```python
from build123d import *
from OCP.BRepAlgoAPI import BRepAlgoAPI_Cut
from OCP.TopTools import TopTools_ListOfShape

# Parameters (mm, degrees)
SKETCH1_W               = 193.19
SKETCH1_H               = 93.85
BOSS_EXTRUDE1_DEPTH     = 32.179999902
SKETCH3_W               = 93.85
SKETCH3_H               = 28.999999912
CUT_EXTRUDE1_DEPTH      = 27.67
SKETCH5_W               = 137.85
SKETCH5_H               = 32.179999902
BOSS_EXTRUDE2_DEPTH     = 12.5
SKETCH6_W               = 32
SKETCH6_H               = 40
CUT_EXTRUDE2_DEPTH      = 118.887561022
SKETCH21_W              = 116.85
SKETCH21_H              = 73.85
CUT_EXTRUDE3_DEPTH      = 118.887561022
CUT_EXTRUDE5_DEPTH      = 118.887561022
CUT_EXTRUDE5_DEPTH_BACK = 29
SKETCH22_W              = 130.49
SKETCH22_H              = 91.75
SKETCH23_W              = 130.49
SKETCH23_H              = 3.18
BOSS_EXTRUDE4_DEPTH     = 6.35
SKETCH25_R              = 2.185
CUT_EXTRUDE6_DEPTH      = 118.887561022
SKETCH26_R              = 2.185
CUT_EXTRUDE8_DEPTH      = 179.78409722
FILLET3_R               = 1
FILLET1_R               = 7.75
FILLET2_R               = 10
CUT_EXTRUDE9_REACH      = 149.229
SKETCH47_R              = 3.5
BOSS_EXTRUDE5_DEPTH     = 8
SKETCH48_R              = 3
CUT_EXTRUDE18_DEPTH     = 6
SKETCH49_R              = 3
CUT_EXTRUDE19_DEPTH     = 5
SKETCH51_R              = 3.5
BOSS_EXTRUDE6_DEPTH     = 8
SKETCH52_R              = 3
CUT_EXTRUDE21_DEPTH     = 5
SKETCH53_W              = 25.1
SKETCH53_H              = 21.647882291
SKETCH53_W_2            = 16.257833485
BOSS_EXTRUDE7_DEPTH     = 3.82
FILLET4_DEPTH           = 21.647882291
FILLET4_START           = -51.344578607
FILLET4_2_DEPTH         = 27.019578607
FILLET4_START_2         = 23.245
FILLET4_3_DEPTH         = 20.253781432
FILLET4_START_3         = 21.647882291
FILLET4_4_DEPTH         = 3.995947947
FILLET4_5_DEPTH         = 10.532117611
SKETCH54_W              = 36.508182433
SKETCH54_H              = 14.6
CUT_EXTRUDE24_DEPTH     = 22.649999902
SKETCH55_W              = 81.374829932
SKETCH55_H              = 14.6
CUT_EXTRUDE26_DEPTH     = 18
SKETCH57_W              = 36.508182433
SKETCH57_H              = 14.6
BOSS_EXTRUDE8_DEPTH     = 4.649999902


with BuildPart() as part:
    # Sketch1 → Boss-Extrude1 (new body)
    with BuildSketch(Plane(origin=(0, 0, 0), x_dir=(1, 0, 0), z_dir=(0, 1, 0))):
        Rectangle(SKETCH1_W, SKETCH1_H)
    extrude(amount=BOSS_EXTRUDE1_DEPTH)

    # Sketch3 → Cut-Extrude1 (cut)
    with BuildSketch(Plane.ZY.offset(96.595)):
        with Locations((0, 14.499999956)):
            Rectangle(SKETCH3_W, SKETCH3_H)
    cut_extrude1 = extrude(amount=-CUT_EXTRUDE1_DEPTH, mode=Mode.SUBTRACT)

    # Mirror1: Cut-Extrude1 across plane
    add(cut_extrude1.mirror(Plane(origin=(0, 0, 0), x_dir=(0, 0, 1), z_dir=(1, 0, 0))), mode=Mode.SUBTRACT)

    # Sketch5 → Boss-Extrude2 (add)
    with BuildSketch(Plane(origin=(0, 0, -46.925), x_dir=(-1, 0, 0), z_dir=(0, 0, -1))):
        with Locations((0, 16.089999951)):
            Rectangle(SKETCH5_W, SKETCH5_H)
    extrude(amount=BOSS_EXTRUDE2_DEPTH)

    # Sketch6 → Cut-Extrude2 (cut, through all)
    with BuildSketch(Plane(origin=(0, 32.179999902, 0), x_dir=(1, 0, 0), z_dir=(0, 1, 0))):
        with Locations((0, 34.425)):
            Rectangle(SKETCH6_W, SKETCH6_H)
    extrude(amount=-CUT_EXTRUDE2_DEPTH, mode=Mode.SUBTRACT)

    # Sketch21 → Cut-Extrude3 (cut, through all)
    with BuildSketch(Plane(origin=(0, 32.179999902, 0), x_dir=(1, 0, 0), z_dir=(0, 1, 0))):
        with Locations((0.5, 0)):
            Rectangle(SKETCH21_W, SKETCH21_H)
    extrude(amount=-CUT_EXTRUDE3_DEPTH, mode=Mode.SUBTRACT)

    # Sketch22 → Cut-Extrude5 (cut, two sides: drawn at the far end of the back side and taken through both)
    with BuildSketch(Plane(origin=(0, 32.179999902, 0), x_dir=(1, 0, 0), z_dir=(0, 1, 0)).offset(-CUT_EXTRUDE5_DEPTH_BACK)):
        with Locations((0.5, -1.05)):
            Rectangle(SKETCH22_W, SKETCH22_H)
    extrude(amount=CUT_EXTRUDE5_DEPTH + CUT_EXTRUDE5_DEPTH_BACK, mode=Mode.SUBTRACT)

    # Sketch23 → Boss-Extrude4 (add)
    with BuildSketch(Plane(origin=(0, 3.18, 0), x_dir=(1, 0, 0), z_dir=(0, 1, 0))):
        with Locations((0.5, -45.335)):
            Rectangle(SKETCH23_W, SKETCH23_H)
    extrude(amount=BOSS_EXTRUDE4_DEPTH)

    # Sketch25 → Cut-Extrude6 (cut, through all)
    with BuildSketch(Plane(origin=(0, 32.179999902, 0), x_dir=(1, 0, 0), z_dir=(0, 1, 0))):
        with Locations(Location((-86.285, 36.085, 0), (0, 0, 270))):
            Circle(SKETCH25_R)
        with Locations(Location((-86.285, 11.085, 0), (0, 0, 270))):
            Circle(SKETCH25_R)
        with Locations(Location((-86.285, -11.085, 0), (0, 0, 270))):
            Circle(SKETCH25_R)
        with Locations(Location((-86.285, -36.085, 0), (0, 0, 270))):
            Circle(SKETCH25_R)
    cut_extrude6 = extrude(amount=-CUT_EXTRUDE6_DEPTH, mode=Mode.SUBTRACT)

    # Sketch26 → Cut-Extrude8 (cut, through all)
    with BuildSketch(Plane.ZY.offset(68.925)):
        with Locations((-12.505, 12.7)):
            Circle(SKETCH26_R)
        with Locations((12.495, 12.7)):
            Circle(SKETCH26_R)
    extrude(amount=-CUT_EXTRUDE8_DEPTH, mode=Mode.SUBTRACT)

    # Mirror4: Cut-Extrude6 across plane
    add(cut_extrude6.mirror(Plane(origin=(0.5, 0, 0), x_dir=(0, 0, 1), z_dir=(1, 0, 0))), mode=Mode.SUBTRACT)

    # Fillet3
    fillet3_edges = [part.edges().sort_by_distance(p)[0] for p in [
        (-68.925, 28.999999912, 0),
        (68.925, 28.999999912, 0),
        (-68.925, 30.589999907, -46.925),
        (68.925, 30.589999907, -46.925),
    ]]
    fillet(fillet3_edges, radius=FILLET3_R)

    # Fillet1
    fillet1_edges = [part.edges().sort_by_distance(p)[0] for p in [
        (-16, 1.589999951, -36.925),
        (16, 1.589999951, -36.925),
    ]]
    fillet(fillet1_edges, radius=FILLET1_R)

    # Fillet2
    fillet2_edges = [part.edges().sort_by_distance(p)[0] for p in [
        (68.925, 16.089999951, -59.425),
        (-68.925, 16.089999951, -59.425),
    ]]
    fillet(fillet2_edges, radius=FILLET2_R)

    # Sketch27 → Cut-Extrude9 (cut, up to next)
    with BuildSketch(Plane(origin=(0, 0, -59.425), x_dir=(-1, 0, 0), z_dir=(0, 0, -1)), mode=Mode.PRIVATE) as cut_extrude9_sk1:
        with BuildLine():
            Line((-2, 3.5), (-2, 10))
            ThreePointArc((-2, 10), (0, 12), (2, 10))
            Line((2, 10), (2, 3.5))
            ThreePointArc((2, 3.5), (0, 1.5), (-2, 3.5))
        make_face()
    cut_extrude9_tool1 = extrude(cut_extrude9_sk1.sketch, amount=-CUT_EXTRUDE9_REACH, mode=Mode.PRIVATE) & part.part
    add(cut_extrude9_tool1.solids().sort_by_distance((0, 6.75, -59.425))[0], mode=Mode.SUBTRACT)

    # Sketch47 → Boss-Extrude5 (add)
    with BuildSketch(Plane(origin=(-64.745, 0, 0), x_dir=(0, 0, -1), z_dir=(1, 0, 0))):
        with Locations((27.825, 9.18)):
            Circle(SKETCH47_R)
    extrude(amount=-BOSS_EXTRUDE5_DEPTH)

    # Sketch48 → Cut-Extrude18 (cut)
    with BuildSketch(Plane(origin=(-64.745, 0, 0), x_dir=(0, 0, -1), z_dir=(1, 0, 0))):
        with Locations((27.825, 9.18)):
            Circle(SKETCH48_R)
    extrude(amount=-CUT_EXTRUDE18_DEPTH, mode=Mode.SUBTRACT)

    # Sketch49 → Cut-Extrude19 (cut)
    with BuildSketch(Plane.XY.offset(-44.825)):
        with Locations((-47.745, 9.18)):
            Circle(SKETCH49_R)
    extrude(amount=-CUT_EXTRUDE19_DEPTH, mode=Mode.SUBTRACT)

    # Sketch51 → Boss-Extrude6 (add)
    with BuildSketch(Plane(origin=(-64.745, 0, 0), x_dir=(0, 0, -1), z_dir=(1, 0, 0))):
        with Locations((-26.745, 9.18)):
            Circle(SKETCH51_R)
    extrude(amount=-BOSS_EXTRUDE6_DEPTH)

    # Sketch52 → Cut-Extrude21 (cut)
    with BuildSketch(Plane(origin=(-64.745, 0, 0), x_dir=(0, 0, -1), z_dir=(1, 0, 0))):
        with Locations((-26.745, 9.18)):
            Circle(SKETCH52_R)
    extrude(amount=-CUT_EXTRUDE21_DEPTH, mode=Mode.SUBTRACT)

    # Sketch53 → Boss-Extrude7 (add)
    with BuildSketch(Plane.ZY.offset(68.925)):
        with Locations((-36.875, 10.823941146)):
            Rectangle(SKETCH53_W, SKETCH53_H)
        with Locations((31.373916743, 10.823941146)):
            Rectangle(SKETCH53_W_2, SKETCH53_H)
    extrude(amount=BOSS_EXTRUDE7_DEPTH)


with BuildPart() as fillet4_tool:
    # Fillet4: read off the stored shape, not the designer's step
    # Fillet4 outline → Fillet4 (new body)
    with BuildSketch(Plane(origin=(0, 0, 0), x_dir=(1, 0, 0), z_dir=(0, 1, 0))):
        with BuildLine():
            Line((-68.925, -39.502833485), (-72.745, -39.502833485))
            ThreePointArc((-72.745, -39.502833485), (-70.033633541, -40.73472644), (-68.925, -43.498781432))
            Line((-68.925, -43.498781432), (-68.925, -39.502833485))
        make_face()
        with BuildLine():
            Line((-72.341407865, 49.425), (-68.925, 49.425))
            ThreePointArc((-68.925, 49.425), (-68.820238369, 50.868695821), (-68.508148475, 52.282142857))
            ThreePointArc((-68.508148475, 52.282142857), (-69.950950646, 50.217865097), (-72.341407865, 49.425))
        make_face()
    extrude(amount=FILLET4_DEPTH)


with BuildPart() as part_1:
    add(part.part)


with BuildPart() as part_2:
    # Fillet4: joined with fillet4_tool
    add(part_1.part.fuse(fillet4_tool.part, tol=0.00001))


with BuildPart() as fillet4_2_tool:
    # Fillet4 2 outline → Fillet4 2 (new body)
    with BuildSketch(Plane.XY.offset(FILLET4_START)):
        with BuildLine():
            ThreePointArc((-68.925, 25.643830238), (-70.033633541, 22.879775246), (-72.745, 21.647882291))
            Line((-72.745, 21.647882291), (-68.925, 21.647882291))
            Line((-68.925, 21.647882291), (-68.925, 25.643830238))
        make_face()
    extrude(amount=FILLET4_2_DEPTH)


with BuildPart() as part_3:
    add(part_2.part)


with BuildPart() as part_4:
    # Fillet4 2: joined with fillet4_2_tool
    add(part_3.part.fuse(fillet4_2_tool.part, tol=0.00001))


with BuildPart() as fillet4_3_tool:
    # Fillet4 3 outline → Fillet4 3 (new body)
    with BuildSketch(Plane.XY.offset(FILLET4_START_2)):
        with BuildLine():
            ThreePointArc((-68.925, 25.643830238), (-70.033633541, 22.879775246), (-72.745, 21.647882291))
            Line((-72.745, 21.647882291), (-68.925, 21.647882291))
            Line((-68.925, 21.647882291), (-68.925, 25.643830238))
        make_face()
    extrude(amount=FILLET4_3_DEPTH)


with BuildPart() as part_5:
    add(part_4.part)


with BuildPart() as part_6:
    # Fillet4 3: joined with fillet4_3_tool
    add(part_5.part.fuse(fillet4_3_tool.part, tol=0.00001))


with BuildPart() as fillet4_4_tool:
    # Fillet4 4 outline → Fillet4 4 (new body)
    with BuildSketch(Plane(origin=(0, 0, 0), x_dir=(1, 0, 0), z_dir=(0, 1, 0)).offset(FILLET4_START_3)):
        with BuildLine():
            ThreePointArc((-68.925, -43.498781432), (-70.033633541, -40.73472644), (-72.745, -39.502833485))
            Line((-72.745, -39.502833485), (-72.745, -43.498781432))
            Line((-72.745, -43.498781432), (-68.925, -43.498781432))
        make_face()
        with BuildLine():
            Line((-68.925, 51.344577615), (-72.745, 51.344578607))
            Line((-72.745, 51.344578607), (-72.745, 49.425))
            Line((-72.745, 49.425), (-72.341407865, 49.425))
            ThreePointArc((-72.341407865, 49.425), (-70.38203163, 49.93775972), (-68.925, 51.344577615))
        make_face()
    extrude(amount=FILLET4_4_DEPTH)


with BuildPart() as part_7:
    add(part_6.part)

    # Fillet4 4: cut by fillet4_4_tool, with a tolerance
    fillet4_4_stock = TopTools_ListOfShape()
    fillet4_4_stock.Append(part_7.part.wrapped)
    fillet4_4_tools = TopTools_ListOfShape()
    fillet4_4_tools.Append(fillet4_4_tool.part.wrapped)
    fillet4_4_cut = BRepAlgoAPI_Cut()
    fillet4_4_cut.SetArguments(fillet4_4_stock)
    fillet4_4_cut.SetTools(fillet4_4_tools)
    fillet4_4_cut.SetFuzzyValue(0.00001)
    fillet4_4_cut.Build()
    add(Compound.cast(fillet4_4_cut.Shape()).solids(), mode=Mode.REPLACE)


with BuildPart() as fillet4_5_tool:
    # Fillet4 5 outline → Fillet4 5 (new body)
    with BuildSketch(Plane(origin=(0, 0, 0), x_dir=(1, 0, 0), z_dir=(0, 1, 0)).offset(FILLET4_START_3)):
        with BuildLine():
            ThreePointArc((-68.508148475, 52.282142857), (-68.686387212, 51.799938762), (-68.925, 51.344577615))
            Line((-68.925, 51.344577615), (-68.925, 49.425))
            ThreePointArc((-68.925, 49.425), (-68.820238369, 50.868695821), (-68.508148475, 52.282142857))
        make_face()
    extrude(amount=FILLET4_5_DEPTH)


with BuildPart() as part_8:
    add(part_7.part)


with BuildPart() as part_9:
    # Fillet4 5: joined with fillet4_5_tool
    add(part_8.part.fuse(fillet4_5_tool.part, tol=0.00001))

    # Sketch54 → Cut-Extrude24 (cut)
    with BuildSketch(Plane(origin=(0, 32.179999902, 0), x_dir=(1, 0, 0), z_dir=(0, 1, 0))):
        with Locations((40.670908784, 52.125)):
            Rectangle(SKETCH54_W, SKETCH54_H)
    extrude(amount=-CUT_EXTRUDE24_DEPTH, mode=Mode.SUBTRACT)

    # Sketch55 → Cut-Extrude26 (cut)
    with BuildSketch(Plane(origin=(0, 32.179999902, 0), x_dir=(1, 0, 0), z_dir=(0, 1, 0))):
        with Locations((-18.270597399, 52.125)):
            Rectangle(SKETCH55_W, SKETCH55_H)
    extrude(amount=-CUT_EXTRUDE26_DEPTH, mode=Mode.SUBTRACT)

    # Sketch57 → Boss-Extrude8 (add)
    with BuildSketch(Plane(origin=(0, 9.53, 0), x_dir=(1, 0, 0), z_dir=(0, 1, 0))):
        with Locations((40.670908784, 52.125)):
            Rectangle(SKETCH57_W, SKETCH57_H)
    extrude(amount=BOSS_EXTRUDE8_DEPTH)


solid = part_9.part
```
Work out the finished part from the listing and answer in its coordinate system (mm). A direction names the side the tool comes from. Coordinates: 2 decimals unless noted, no trailing zeros. Write each loop counter-clockwise with the first axis right and the second up, starting at its lowest first coordinate (ties: lowest second). Pieces come first, ordered by that corner, then holes.
Q1. A cutting plane is placed at B-B, the plane x = 49. Give the vertices of the cut face in (y, z) (3 decimals).
Q2. A cutting plane is placed at A-A, the plane z = 16.5. Give the vertices of the cut face in (x, y) (3 decimals).
Q3. Which of the six approach directions +Z, -Z, +X, -X, +Y, -Y give full straight-line access (tool end or side, diameter ignored) to faces 1 (the face through (-71, 13, 23.245)), 2 (the face through (-50.742, 9.312, -47.29)), 3 (the face through (-16, 7, -49))?
Q4. A cutting plane is placed at D-D, the plane z = -28. Give the vertices of the cut face in (x, y) (3 decimals), then the cut area to 3 significant figures.
Q5. Find the intervals of material crossed by line 1 (Z direction, x = 11.5, y = 2) (3 decimals); line 2 (Z direction, x = 39.5, y = 2) (3 decimals); line 3 (Z direction, x = -68, y = 9) (3 decimals), in increasing order.
Q6. Each of these flat-tipped pins is pushed along its axis until it touches: pin 1 Ø1.6 at (x, y) = (-89.5, 31) entering from -Z (3 decimals); pin 2 Ø6 at (y, z) = (22.5, 27.5) entering from +X (3 decimals); pin 3 Ø5.5 at (y, z) = (6, -57) entering from +X; pin 4 Ø10 at (x, z) = (-76, 33) entering from -Y. Where does it stop, or does it pass through?
Q7. A cutting plane is placed at C-C, the plane y = 19.5. Give the vertices of the cut face in (x, z) (3 decimals).
Q8. Determine the mould class of faces 4 (the face through (-17, 0, -42)), 5 (the face through (-64.829, 16.315, -57.496)), 6 (the face through (-71, 13, -24.325)) for opening direction Z: released by +Z, released by -Z, zero draft, split by the parting line, or undercut.
Findings below:
1. outline: (0, -59.425) - (14.18, -59.425) - (14.18, -44.825) - (3.18, -44.825) - (3.18, -36.925) - (0, -36.925) - close; (0, 36.925) - (3.18, 36.925) - (3.18, 43.745) - (9.53, 43.745) - (9.53, 46.925) - (0, 46.925) - close
2. outline: (-96.595, 29) - (-69.925, 29) arc R1 cw to (-68.925, 28) - (-68.925, 0) - (-57.925, 0) - (-57.925, 3.18) - (-64.745, 3.18) - (-64.745, 32.18) - (-96.595, 32.18) - close; (58.925, 0) - (68.925, 0) - (68.925, 28) arc R1 cw to (69.925, 29) - (96.595, 29) - (96.595, 32.18) - (65.745, 32.18) - (65.745, 3.18) - (58.925, 3.18) - close
3. face 1: -X, -Y
3. face 2: none
3. face 3: +Y, -Y
4. outline: (-96.595, 29) - (-69.925, 29) arc R1 cw to (-68.925, 28) - (-68.925, 25.644) arc R4 cw to (-72.745, 21.648) - (-72.745, 0) - (-57.925, 0) - (-57.925, 3.18) - (-64.745, 3.18) - (-64.745, 6.185) - (-68.925, 6.185) - (-68.925, 12.175) - (-64.745, 12.175) - (-64.745, 32.18) - (-96.595, 32.18) - close; (58.925, 0) - (68.925, 0) - (68.925, 28) arc R1 cw to (69.925, 29) - (96.595, 29) - (96.595, 32.18) - (65.745, 32.18) - (65.745, 3.18) - (58.925, 3.18) - close
4. area: 518 mm2
5. line 1: z = -59.425 to -54.425, 36.925 to 46.925
5. line 2: z = -59.425 to -36.925, 36.925 to 46.925
5. line 3: z = -53.626 to -30.82, -24.83 to 23.75, 29.74 to 46.925
6. pin 1: stops at z = -46.925
6. pin 2: stops at x = 68.925
6. pin 3: stops at x = 67.68
6. pin 4: stops at y = 0
7. outline: (-72.745, -49.425) - (-72.341, -49.425) arc R4 cw to (-68.508, -52.282) arc R10 ccw to (-58.958, -59.425) - (-58.958, -44.825) - (-64.745, -44.825) - (-64.745, 46.925) - (-68.925, 46.925) - (-68.925, 43.499) arc R4 cw to (-72.745, 39.503) - (-72.745, 23.245) - (-68.925, 23.245) - (-68.925, -24.325) - (-72.745, -24.325) - close; (58.925, -59.425) arc R10 ccw to (68.925, -49.425) - (68.925, 46.925) - (65.745, 46.925) - (65.745, -44.825) - (58.925, -44.825) - close
8. face 4: zero draft
8. face 5: released by -Z
8. face 6: undercut
